Autodesk Inventor part; units mm, degrees
ref_plane "Work Plane1" through (0, 9.25, 10) normal (0, 0, 1) x (1, 0, 0)
ref_plane "YZ Plane" through (0, 0, 0) normal (1, 0, 0) x (0, 1, 0)
ref_plane "XZ Plane" through (0, 0, 0) normal (0, 1, 0) x (-1, 0, 0)
sketch "Sketch1" plane through (0, 0, 0) normal (0, 0, 1) x (1, 0, 0)
  line L0 (0, -3.1) -> (0, 18.6) construction
  line L1 (-2, 0) -> (12, 0) construction
  line L2 (9, 0) -> (9, 3)
  line L3 (9, 3) -> (10, 3)
  line L4 (10, 3) -> (10, 15.5)
  line L5 (10, 15.5) -> (0, 15.5)
  line L6 (0, 15.5) -> (0, 12)
  line L7 (0, 12) -> (3, 12)
  line L8 (3, 12) -> (3, 3)
  line L9 (3, 3) -> (7.5, 3)
  line L10 (7.5, 3) -> (7.5, 0)
  line L11 (7.5, 0) -> (9, 0)
  point P0 (0, 0)
  point P1 (3, 7.5)
  dimension "d0" = 15.5
  dimension "d1" = 12
  dimension "d2" = 3
  dimension "d4" = 6
  dimension "d5" = 15
  dimension "d6" = 18
  dimension "d7" = 20
revolve "Revolution1" add sketch "Sketch1" angle 360 about axis through (0, -10, 0) along (0, 1, 0)
fillet "Fillet1" radius 1.2 1 edges at (-10, 15.5, 0)
ref_plane "Work Plane1" through (0, 9.25, 10) normal (0, 0, 1) x (1, 0, 0)
sketch "Sketch3" plane through (0, 9.25, 10) normal (0, 0, 1) x (1, 0, 0)
  line L0 (9, -9.25) -> (-9, -9.25) construction
  line L1 (0, -12.35) -> (0, 9.35) construction
  point P0 (0, -9.25)
  point P1 (0, -2.85)
  dimension "d11" = 6.4
hole "Hole1" at (0, 6.4, 10) direction (0, 0, -1) diameter 3.242 end up to surface counterbore diameter 5.75 counterbore depth 1.5
properties part number "encoder_cap"
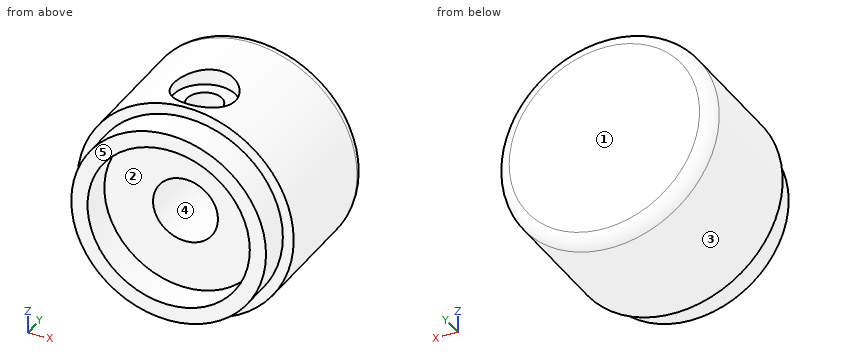
Can you work these out from the model? Positions are in its coordinate system, mm. Face numbers are marked on the shaded views. A direction names the side the tool comes from. Coordinates: 2 decimals unless noted, no trailing zeros. Loops run counter-clockwise (first coordinate to the right, second up) from the corner with the lowest first, then second, coordinate; pieces in that order, holes last. Notation, with made-up numbers: (86.25, -27.5) -> (120.25, -27.5) arc R23 cw to (120.25, -11.5) -> close; hole circle Ø8 at (73, -9). An arc over 180 degrees is marked (long way). Put each result on its own line as item: value. Start each with the question number.
Q1. I want a section at C-C (y = 10.75). Write out the boundary of the cut face in (x, z).
Q2. I want a section at D-D (y = 12.5). Write out the boundary of the cut face in (x, z).
Q3. For the marked faces 1 and 2, which set-ups out of +Z, -Z, +X, -X, +Y, -Y let a thin tool reach every point of the face, with its end or its side?
Q4. Thinking about a two-plate mould opening in Z: for the marked faces 3, 4 and 5, which applies, pulls with the +Z half, pulls with the -Z half, needs draft (parallel to the pull), parting line crosses it, or undercut?
Q5. I'm going to push flat-ended pins straight in: P1, Ø8, axis at y = 7.5, z = -7, coming from the -X side; P2, Ø3, axis at x = 0.5, z = -1, coming from the -Y side; P3, Ø3, axis at y = 12, z = 5, coming from the -X side. Where does each tip first touch, or does it pass through?
Q6. If I drill on line 1 (Z direction, x = 0, y = 1.5); line 2 (Y direction, x = 0, z = 3.95); line 3 (X direction, y = 5, z = 0), over which ranges is the centre line in solid material (lowest first)? Write a range as [from, to].
Q7. I want a section at B-B (z = 0). Write out the boundary of the cut face in (x, y).
Q8. I want a section at A-A (x = 0). Write out the boundary of the cut face in (y, z) (3 decimals).
Taken from the geometry:
1. outline: circle Ø20 at (0, 0); hole circle Ø6 at (0, 0)
2. outline: circle Ø20 at (0, 0)
3. face 1: +Z, -Z, +X, -X, +Y
3. face 2: -Y
4. face 3: parting line crosses it
4. face 4: undercut
4. face 5: needs draft
5. P1: stops at x = -9.54
5. P2: stops at y = 12
5. P3: stops at x = -9.37
6. line 1: z = [-9, -7.5], [7.5, 9]
6. line 2: y = [3, 4.78], [8.02, 15.5]
6. line 3: x = [-10, -3], [3, 10]
7. outline: (-10, 3) -> (-9, 3) -> (-9, 0) -> (-7.5, 0) -> (-7.5, 3) -> (-3, 3) -> (-3, 12) -> (3, 12) -> (3, 3) -> (7.5, 3) -> (7.5, 0) -> (9, 0) -> (9, 3) -> (10, 3) -> (10, 14.3) arc R1.2 ccw to (8.8, 15.5) -> (-8.8, 15.5) arc R1.2 ccw to (-10, 14.3) -> close
8. outline: (0, -9) -> (3, -9) -> (3, -10) -> (14.3, -10) arc R1.2 ccw to (15.5, -8.8) -> (15.5, 8.8) arc R1.2 ccw to (14.3, 10) -> (9.275, 10) -> (9.275, 8.5) -> (8.021, 8.5) -> (8.021, 3) -> (12, 3) -> (12, -3) -> (3, -3) -> (3, -7.5) -> (0, -7.5) -> close; (0, 7.5) -> (3, 7.5) -> (3, 3) -> (4.779, 3) -> (4.779, 8.5) -> (3.525, 8.5) -> (3.525, 10) -> (3, 10) -> (3, 9) -> (0, 9) -> close
